Answer from the drawing. Dimensions are ordinates in mm from the lowest x, y and z of the part. A direction names the side the tool comes from. Round coordinates to 2 decimals unless told otherwise and drop trailing zeros. Loops run counter-clockwise (first coordinate to the right, second up) from the corner with the lowest first, then second, coordinate; pieces in that order, holes last. Notation, with made-up numbers: M 50,43 L 81,43 A15 ccw 81,56 Z; hole C 56,75.5 d1. An arc over 180 degrees is marked long. Answer as CSV lines item,"result".
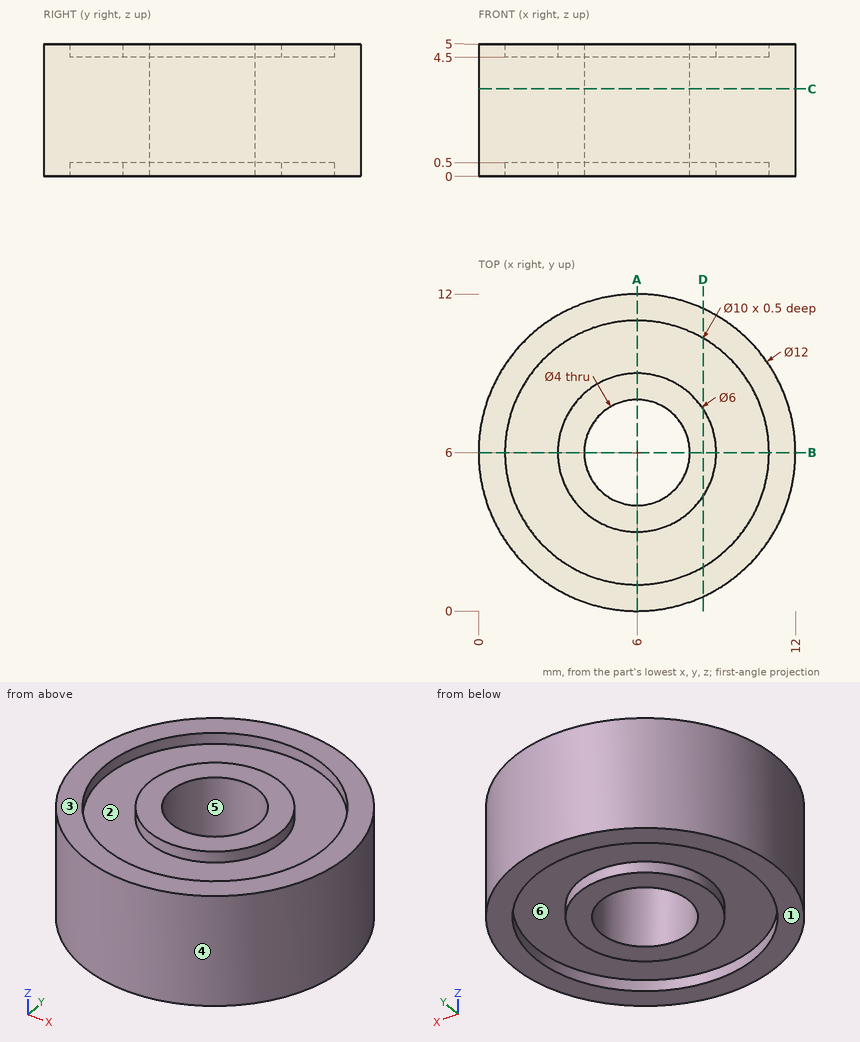
1) This flat-tipped pin is pushed along its axis until it touches: P1, Ø3, axis at y = 2, z = 1.5, coming from the +X side. Where does it stop, or does it pass through?
Evaluation:
P1,"stops at x = 11.45"
2) Find section C-C, the plane z = 3.3. Give the vertices of the cut face in (x, y).
Evaluation:
outline,"C 6,6 d12; hole C 6,6 d4"
3) Find section A-A, the plane x = 6. Give the vertices of the cut face in (y, z).
Evaluation:
outline,"M 0,0 L 1,0 L 1,0.5 L 3,0.5 L 3,0 L 4,0 L 4,5 L 3,5 L 3,4.5 L 1,4.5 L 1,5 L 0,5 Z; M 8,0 L 9,0 L 9,0.5 L 11,0.5 L 11,0 L 12,0 L 12,5 L 11,5 L 11,4.5 L 9,4.5 L 9,5 L 8,5 Z"
4) Determine the mould class of the marked faces 3, 4, 5 and 6 for opening direction Y: released by +Y, released by -Y, zero draft, split by the parting line, or undercut.
Evaluation:
face 3,"zero draft"
face 4,"split by the parting line"
face 5,"undercut"
face 6,"undercut"
5) A tool of negligible diameter and unlimited length cuts with its end or side. For the marked faces 1 and 2, from which of +Z, -Z, +X, -X, +Y, -Y can it reach the whole face along a straight path? Write none if from no direction.
Evaluation:
face 1,"-Z, +X, -X, +Y, -Y"
face 2,"+Z"
6) Straight lines are drawn through the part: line 1 (Y direction, x = 6, z = 4.85); line 2 (Y direction, x = 6, z = 1.2); line 3 (Y direction, x = 5, z = 4.25). For each, find the intervals that lie inside material, in ascending order.
Evaluation:
line 1,"y = 0 to 1, 3 to 4, 8 to 9, 11 to 12"
line 2,"y = 0 to 4, 8 to 12"
line 3,"y = 0.08 to 4.27, 7.73 to 11.92"
7) Find section D-D, the plane x = 8.5. Give the vertices of the cut face in (y, z), then the cut area to 3 significant figures.
Evaluation:
outline,"M 0.55,0 L 1.67,0 L 1.67,0.5 L 4.34,0.5 L 4.34,0 L 7.66,0 L 7.66,0.5 L 10.33,0.5 L 10.33,0 L 11.45,0 L 11.45,5 L 10.33,5 L 10.33,4.5 L 7.66,4.5 L 7.66,5 L 4.34,5 L 4.34,4.5 L 1.67,4.5 L 1.67,5 L 0.55,5 Z"
area,"49.2 mm^2"
